Work out the finished part from the listing and answer in its coordinate system (mm). Face numbers are marked on the shaded views. A direction names the side the tool comes from. Coordinates: 2 decimals unless noted, no trailing zeros. Loops run counter-clockwise (first coordinate to the right, second up) from the corner with the lowest first, then second, coordinate; pieces in that order, holes last. Notation, with made-up numbers: (-2.75, 54.5) - (48.25, 54.5) arc R21 ccw to (48.25, 85.5) - close; hole circle Ø8 at (74, 17.25). An arc over 180 degrees is marked (long way). Write each question's results on one line, items separated by ' | '. Start each with the question number.
Item 1: A tool of negligible diameter and unlimited length cuts with its end or side. For the marked faces 1 and 2, from which of +Z, -Z, +X, -X, +Y, -Y can it reach the whole face along a straight path? Write none if from no direction.
Item 2: Consider probe 1 along X at (y, z) = (3.5, 0); probe 2 along X at (y, z) = (5.2, 0). Determine where each line is inside the solid, lowest interval first. Write a range as [from, to].
Item 3: Section D-D, the plane y = 8.5 is taken. Write down the section's boundary in (x, z), plus the area to 3 significant figures.
Item 4: Section A-A, the plane x = 0 is taken. Count the separate pieces of the cut face and the enclosed holes in it, plus the area to 3 significant figures.
Item 5: Section C-C, the plane y = 1.25 is taken. Write down the section's boundary in (x, z).
Item 6: For a pull along Z with two mould halves and no side action, classify the marked faces 3, 4 and 5 as +Z half, -Z half, draft (parallel to the pull), parting line (faces both ways), or undercut.
Item 7: Each of these flat-tipped pins is pushed along its axis until it touches: pin 1 Ø6 at (y, z) = (3, -5) entering from -X; pin 2 Ø2 at (y, z) = (3, -10) entering from -X; pin 3 Ø6 at (y, z) = (8, -1) entering from -X; pin 4 Ø7 at (x, z) = (-1, 3) entering from +Y. Where does it stop, or does it pass through?
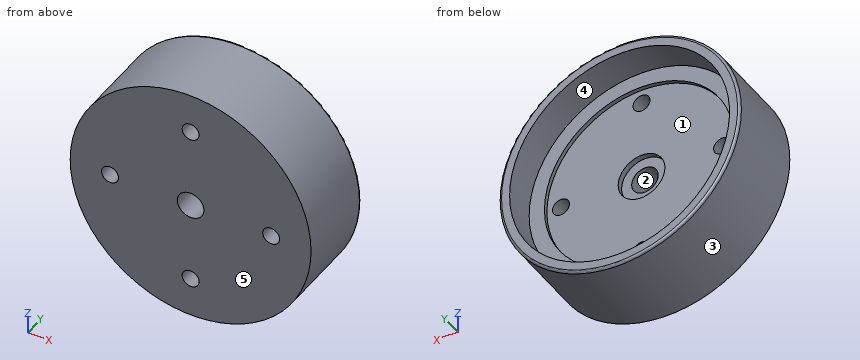
from build123d import *

# Parameters (mm, degrees)
SKETCH1_R           = 14.95
BOSS_EXTRUDE1_DEPTH = 6.2
SKETCH2_R           = 11.75
CUT_EXTRUDE1_DEPTH  = 0.5
SKETCH3_R           = 14.95
SKETCH3_R_2         = 13.65
BOSS_EXTRUDE2_DEPTH = 4
FILLET1_R           = 0.3
SKETCH4_R           = 1.65
CUT_EXTRUDE2_DEPTH  = 6.7
SKETCH18_R          = 2.9
CUT_EXTRUDE10_DEPTH = 0.7
SKETCH19_R          = 1.05
CUT_EXTRUDE11_DEPTH = 6.7


with BuildPart() as part:
    # Sketch1 → Boss-Extrude1 (new body)
    with BuildSketch(Plane(origin=(0, 0, 0), x_dir=(1, 0, 0), z_dir=(0, 1, 0))):
        Circle(SKETCH1_R)
    extrude(amount=BOSS_EXTRUDE1_DEPTH)

    # Sketch2 → Cut-Extrude1 (cut)
    with BuildSketch(Plane(origin=(0, 6.2, 0), x_dir=(1, 0, 0), z_dir=(0, 1, 0))):
        Circle(SKETCH2_R)
    extrude(amount=-CUT_EXTRUDE1_DEPTH, mode=Mode.SUBTRACT)

    # Sketch3 → Boss-Extrude2 (add)
    with BuildSketch(Plane(origin=(0, 6.2, 0), x_dir=(1, 0, 0), z_dir=(0, 1, 0))):
        Circle(SKETCH3_R)
        Circle(SKETCH3_R_2, mode=Mode.SUBTRACT)
    extrude(amount=BOSS_EXTRUDE2_DEPTH)

    # Fillet1
    fillet1_edges = [part.edges().sort_by_distance(p)[0] for p in [
        (-14.95, 10.2, 0),
    ]]
    fillet(fillet1_edges, radius=FILLET1_R)

    # Sketch4 → Cut-Extrude2 (cut, through all)
    with BuildSketch(Plane(origin=(0, 5.7, 0), x_dir=(1, 0, 0), z_dir=(0, 1, 0))):
        Circle(SKETCH4_R)
    extrude(amount=-CUT_EXTRUDE2_DEPTH, mode=Mode.SUBTRACT)

    # Sketch18 → Cut-Extrude10 (cut)
    with BuildSketch(Plane(origin=(0, 5.7, 0), x_dir=(1, 0, 0), z_dir=(0, 1, 0))):
        Circle(SKETCH18_R)
    extrude(amount=-CUT_EXTRUDE10_DEPTH, mode=Mode.SUBTRACT)

    # Sketch19 → Cut-Extrude11 (cut, through all)
    with BuildSketch(Plane(origin=(0, 5.7, 0), x_dir=(1, 0, 0), z_dir=(0, 1, 0))):
        with Locations((0, 10)):
            Circle(SKETCH19_R)
        with Locations((10, 0)):
            Circle(SKETCH19_R)
        with Locations((0, -10)):
            Circle(SKETCH19_R)
        with Locations((-10, 0)):
            Circle(SKETCH19_R)
    extrude(amount=-CUT_EXTRUDE11_DEPTH, mode=Mode.SUBTRACT)


solid = part.part
Answer key:
1) face 1: +Y | face 2: +Y, -Y
2) probe 1: x = [-14.95, -11.05], [-8.95, -1.65], [1.65, 8.95], [11.05, 14.95] | probe 2: x = [-14.95, -11.05], [-8.95, -2.9], [2.9, 8.95], [11.05, 14.95]
3) outline: circle Ø29.9 at (0, 0); hole circle Ø27.3 at (0, 0) | area: 117 mm^2
4) separate pieces: 4 | enclosed holes: 0 | area: 139 mm^2
5) outline: circle Ø29.9 at (0, 0); hole circle Ø2.1 at (-10, 0); hole circle Ø3.3 at (0, 0); hole circle Ø2.1 at (0, -10); hole circle Ø2.1 at (0, 10); hole circle Ø2.1 at (10, 0)
6) face 3: parting line | face 4: undercut | face 5: draft
7) pin 1: stops at x = -14.82 | pin 2: stops at x = -11.94 | pin 3: stops at x = -14.95 | pin 4: stops at y = 5.7
